The model under review builds one solid part; all positions refer to its coordinate system, in mm. Face numbers are marked on the shaded views. A direction names the side the tool comes from. Give positions to 0.01 mm unless a question says otherwise; leave off trailing zeros. Order: outer loops, then holes, each group sorted by start corner. A loop starts at its lowest first (then second) coordinate and runs counter-clockwise, first axis right, second up. Notation, with made-up numbers: (18, 50.25) -> (44, 50.25) arc R14 ccw to (44, 59.25) -> close; hole circle Ø7 at (51.5, 55.5). An arc over 180 degrees is marked (long way). Answer as a JSON object with one key per item and string values. Group by question number.
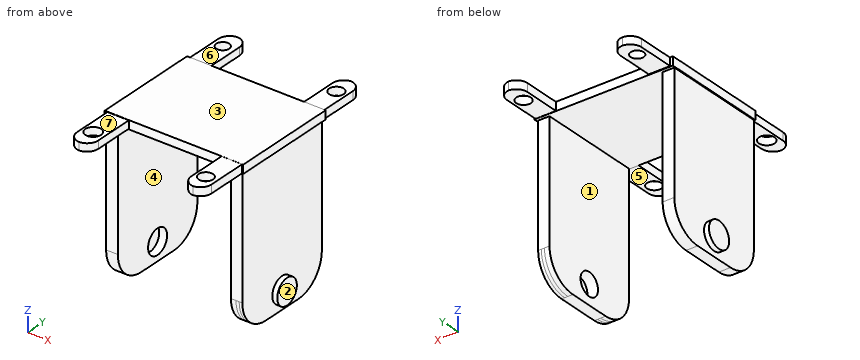
from build123d import *

# Parameters (mm, degrees)
F0_W         = 77.900249511
F0_H         = 6.2239915133
F1_DEPTH     = 50.292
F2_W         = 5.9690438211
F2_H         = 109.3528494239
F2_W_2       = 6.2078051269
F2_H_2       = 109.8303757608
F3_DEPTH     = 37.592
F4_R         = 22.0755688143
F5_DEPTH     = 2.286
F7_R         = 9.5028337992
F8_DEPTH     = 3.6
F6_R         = 9.2619968466
F9_DEPTH     = 3.6
F10_R        = 8.2457773543
F12_DEPTH    = 7.7
F11_R        = 8.9872233932
F13_DEPTH    = 5.7
F14_W        = 14.8572660983
F14_H        = 6.0232169926
F14_W_2      = 15.4595859349
F14_H_2      = 5.6216679513
F15_DEPTH    = 75
F16_T1_DEPTH = 46.6632985117
F16_T3_DEPTH = 47.064847553
F17_R        = 4.7067592452
F17_R_2      = 5.2876360091
F17_R_3      = 5.6910023403
F17_R_4      = 5.1821036644
F18_DEPTH    = 25


# Not quite as in the source:
# - a fillet or chamfer that OpenCascade refuses, or shapes differently, is made with other operations: its cross-section is extruded or revolved along the edge and cut away or added


with BuildPart() as f1:
    # F0 (on Right) → F1 (new body, symmetric)
    with BuildSketch(Plane.YZ):
        with Locations((0.9574238211, 36.620259285)):
            Rectangle(F0_W, F0_H)
    extrude(amount=F1_DEPTH, both=True)

    # F2 (on Front) → F3 (join, symmetric)
    with BuildSketch(Plane.XZ):
        with Locations((44.0515298396, -20.6528864801)):
            Rectangle(F2_W, F2_H)
        with Locations((-44.1709104925, -20.4141233116)):
            Rectangle(F2_W_2, F2_H_2)
    extrude(amount=F3_DEPTH, both=True)

    # F4
    f4_edges = [f1.edges().sort_by_distance(p)[0] for p in [
        (44.05153, 37.592, -75.329311),
        (44.05153, -37.592, -75.329311),
        (-44.17091, -37.592, -75.329311),
        (-44.17091, 37.592, -75.329311),
    ]]
    fillet(f4_edges, radius=F4_R)

    # F5 (add, symmetric): faces of the model
    f5_faces = [f1.faces().sort_by_distance(p)[0] for p in [
        (47.0360517502, 0, -19.6123684117),
        (-47.274813056, 0, -19.6123684117),
    ]]
    extrude(f5_faces, amount=F5_DEPTH, both=True, dir=(1, 0, 0))

    # F7 (on face) → F8 (join)
    with BuildSketch(Plane(origin=(-49.560813056, 0, 0), x_dir=(0, -1, 0), z_dir=(-1, 0, 0))):
        with Locations((0, -61.9606114924)):
            Circle(F7_R)
    extrude(amount=F8_DEPTH)

    # F6 (on face) → F9 (join)
    with BuildSketch(Plane.YZ.offset(49.3220517502)):
        with Locations((0, -61.9290173054)):
            Circle(F6_R)
    extrude(amount=F9_DEPTH)

    # F10 (on face) → F12 (cut)
    with BuildSketch(Plane(origin=(41.0670079291, 0, 0), x_dir=(0, -1, 0), z_dir=(-1, 0, 0))):
        with Locations((0, -61.2058117986)):
            Circle(F10_R)
    extrude(amount=-F12_DEPTH, mode=Mode.SUBTRACT)

    # F11 (on face) → F13 (cut)
    with BuildSketch(Plane.YZ.offset(-41.0670079291)):
        with Locations((0, -62.1923357248)):
            Circle(F11_R)
    extrude(amount=-F13_DEPTH, mode=Mode.SUBTRACT)

    # F14 (on Front) → F15 (join, symmetric)
    with BuildSketch(Plane.XZ):
        with Locations((42.047848925, 36.6818103939)):
            Rectangle(F14_W, F14_H)
        with Locations((-40.5197497457, 36.7389488965)):
            Rectangle(F14_W_2, F14_H_2)
    extrude(amount=F15_DEPTH, both=True)

    # F16: fillet of radius 8.2083261121 on 8 edges, made by hand

    # F16_s2 → F16_t1 (cut)
    with BuildSketch(Plane.XY.offset(13.4072996407)):
        with BuildLine():
            ThreePointArc((-32.7899567783, 66.7916738879), (-35.1941198343, 72.595836944), (-40.9982828904, 75))
            Line((-40.9982828904, 75), (-32.7899567783, 75))
            Line((-32.7899567783, 75), (-32.7899567783, 66.7916738879))
        make_face()
        with BuildLine():
            ThreePointArc((-48.2495427132, 66.7916738879), (-45.8453796571, 72.595836944), (-40.0412166011, 75))
            Line((-40.0412166011, 75), (-48.2495427132, 75))
            Line((-48.2495427132, 75), (-48.2495427132, 66.7916738879))
        make_face()
        with BuildLine():
            ThreePointArc((-48.2495427132, -66.7916738879), (-45.8453796571, -72.595836944), (-40.0412166011, -75))
            Line((-40.0412166011, -75), (-48.2495427132, -75))
            Line((-48.2495427132, -75), (-48.2495427132, -66.7916738879))
        make_face()
        with BuildLine():
            ThreePointArc((-32.7899567783, -66.7916738879), (-35.1941198343, -72.595836944), (-40.9982828904, -75))
            Line((-40.9982828904, -75), (-32.7899567783, -75))
            Line((-32.7899567783, -75), (-32.7899567783, -66.7916738879))
        make_face()
    extrude(amount=F16_T1_DEPTH, mode=Mode.SUBTRACT)

    # F16_s4 → F16_t3 (cut)
    with BuildSketch(Plane.XY.offset(13.1493866174)):
        with BuildLine():
            ThreePointArc((49.4764819741, 66.7916738879), (47.0723189181, 72.595836944), (41.2681558621, 75))
            Line((41.2681558621, 75), (49.4764819741, 75))
            Line((49.4764819741, 75), (49.4764819741, 66.7916738879))
        make_face()
        with BuildLine():
            ThreePointArc((34.6192158759, 66.7916738879), (37.0233789319, 72.595836944), (42.8275419879, 75))
            Line((42.8275419879, 75), (34.6192158759, 75))
            Line((34.6192158759, 75), (34.6192158759, 66.7916738879))
        make_face()
        with BuildLine():
            ThreePointArc((49.4764819741, -66.7916738879), (47.0723189181, -72.595836944), (41.2681558621, -75))
            Line((41.2681558621, -75), (49.4764819741, -75))
            Line((49.4764819741, -75), (49.4764819741, -66.7916738879))
        make_face()
        with BuildLine():
            ThreePointArc((34.6192158759, -66.7916738879), (37.0233789319, -72.595836944), (42.8275419879, -75))
            Line((42.8275419879, -75), (34.6192158759, -75))
            Line((34.6192158759, -75), (34.6192158759, -66.7916738879))
        make_face()
    extrude(amount=F16_T3_DEPTH, mode=Mode.SUBTRACT)

    # F17 (on face) → F18 (cut)
    with BuildSketch(Plane.XY.offset(39.6934188902)):
        with Locations((-41.1323793232, 61.7104582489)):
            Circle(F17_R)
        with Locations((42.1323850751, 60.7389695942)):
            Circle(F17_R_2)
        with Locations((-41.0092622042, -60.9235055745)):
            Circle(F17_R_3)
        with Locations((41.5508002043, -61.9366765022)):
            Circle(F17_R_4)
    extrude(amount=-F18_DEPTH, mode=Mode.SUBTRACT)


solid = f1.part
1. Machinability: for the marked faces 4, 5, 6 and 7, which of the approach directions +Z, -Z, +X, -X, +Y, -Y give a long, thin tool a straight path to every point of the face, cutting with its end or side? Answer none if there is none.
2. Take a section at D-D on z = -67. Give the boundary of the cut face in (x, y), plus the area to 3 significant figures.
3. For pin 1 (16.5 mm diameter, centred on x = 41, y = 49, fed in from -Z); pin 2 (12 mm diameter, centred on x = 41, y = 59.5, fed in from +Z); pin 3 (3 mm diameter, centred on y = -15, z = 35.5, fed in from -X), all flat-tipped, find the tip position at first contact; note any pin that passes through.
4. For probe 1 along Z at (x, y) = (-45.15, 0); probe 2 along X at (y, z) = (29.5, -38); probe 3 along Z at (x, y) = (43, 0), list the stretches that pass through material, from the lowest coordinate up. Write a range as [from, to].
5. Take a section at A-A on z = -2. Give the boundary of the cut face in (x, y).
6. Take a section at C-C on x = -29. Give the boundary of the cut face in (y, z), plus the area to 3 significant figures.
7. Draft analysis for pull direction X (two halves, no side actions). For the marked faces 1, 2 and 3, state which applies: pulls with the +X half, pulls with the -X half, needs draft (parallel to the pull), parting line crosses it, or undercut.
8. Take a section at B-B on y = 0. Give the boundary of the cut face in (x, z), plus the area to 3 significant figures.
Checks:
{
 "1": {"face 4": "-Z, +Y, -Y", "face 5": "-Z, +X, -X, -Y", "face 6": "+Z, -X, +Y", "face 7": "+Z, -X, -Y"},
 "2": {"outline": "(-53.16, -8.06) -> (-49.56, -8.06) -> (-49.56, -32.79) -> (-41.07, -32.79) -> (-41.07, -7.59) -> (-46.77, -7.59) -> (-46.77, 7.59) -> (-41.07, 7.59) -> (-41.07, 32.79) -> (-49.56, 32.79) -> (-49.56, 8.06) -> (-53.16, 8.06) -> close; (41.07, -32.79) -> (49.32, -32.79) -> (49.32, -7.75) -> (52.92, -7.75) -> (52.92, 7.75) -> (49.32, 7.75) -> (49.32, 32.79) -> (41.07, 32.79) -> (41.07, 5.87) -> (48.77, 5.87) -> (48.77, -5.87) -> (41.07, -5.87) -> close", "area": "1,040 mm2"},
 "3": {"pin 1": "stops at z = 33.67", "pin 2": "stops at z = 39.69", "pin 3": "stops at x = -50.29"},
 "4": {"probe 1": "z = [-75.33, -71.18], [-53.21, 39.73]", "probe 2": "x = [-49.56, -41.07], [41.07, 49.32]", "probe 3": "z = [-75.33, -69.45], [-52.96, 39.73]"},
 "5": {"outline": "(-49.56, -37.59) -> (-41.07, -37.59) -> (-41.07, 37.59) -> (-49.56, 37.59) -> close; (41.07, -37.59) -> (49.32, -37.59) -> (49.32, 37.59) -> (41.07, 37.59) -> close"},
 "6": {"outline": "(-37.99, 33.51) -> (39.91, 33.51) -> (39.91, 39.73) -> (-37.99, 39.73) -> close", "area": "485 mm2"},
 "7": {"face 1": "undercut", "face 2": "pulls with the +X half", "face 3": "needs draft"},
 "8": {"outline": "(-53.16, -71.46) -> (-49.56, -71.46) -> (-49.56, -75.33) -> (-41.07, -75.33) -> (-41.07, -71.18) -> (-46.77, -71.18) -> (-46.77, -53.21) -> (-41.07, -53.21) -> (-41.07, 33.51) -> (41.07, 33.51) -> (41.07, -52.96) -> (48.77, -52.96) -> (48.77, -69.45) -> (41.07, -69.45) -> (41.07, -75.33) -> (49.32, -75.33) -> (49.32, -71.19) -> (52.92, -71.19) -> (52.92, -52.67) -> (49.32, -52.67) -> (49.32, 33.51) -> (50.29, 33.51) -> (50.29, 39.73) -> (-50.29, 39.73) -> (-50.29, 33.51) -> (-49.56, 33.51) -> (-49.56, -52.46) -> (-53.16, -52.46) -> close", "area": "2,350 mm2"}
}
